CAD build for the part. Positions are in the model's coordinates, mm. Face numbers are marked on the shaded views. A direction names the side the tool comes from. Give positions to 0.01 mm unless a question says otherwise; leave off trailing zeros. Write each loop counter-clockwise with the first axis right and the second up, starting at its lowest first coordinate (ties: lowest second). Pieces come first, ordered by that corner, then holes. Notation, with made-up numbers: (-39.75, 14.25) - (-29.75, 14.25) arc R25 ccw to (-29.75, 47.25) - close; hole circle Ø9 at (-2, 22.5). An arc over 180 degrees is marked (long way). Answer as a JSON object with one key per item and string values.
from build123d import *

# Parameters (mm, degrees)
F1_DEPTH  = 10
F3_DEPTH  = 100
F4_R      = 35
F5_DEPTH  = 90
F6_DEPTH  = 95.001
F7_R      = 5
F10_R     = 4
F11_DEPTH = 18


with BuildPart() as f1:
    # F0 (on Top) → F1 (new body)
    with BuildSketch(Plane.XY):
        Polygon((-6, 61.6815258077), (-6, 41.6815258077), (-37, 41.6815258077), (-37, 29.6815258077), (-28.3371814517, 29.6815258077), (-40, -30.3184741923), (-40, -125.3184741923), (0, -125.3184741923), (40, -125.3184741923), (40, -30.3184741923), (28.3371814517, 29.6815258077), (37, 29.6815258077), (37, 41.6815258077), (6, 41.6815258077), (6, 61.6815258077), (0, 61.6815258077), align=None)
        Polygon((-8.5239209836, -30.3184741923), (-32, -30.3184741923), (-22.8734250069, 16.6336838404), align=None, mode=Mode.SUBTRACT)
        Polygon((-18.3371814517, 29.6815258077), (-6, 29.6815258077), (-6, -10.686231312), align=None, mode=Mode.SUBTRACT)
        Polygon((6, -10.686231312), (6, 29.6815258077), (18.3371814517, 29.6815258077), align=None, mode=Mode.SUBTRACT)
        Polygon((22.8734250069, 16.6336838404), (32, -30.3184741923), (8.5239209836, -30.3184741923), align=None, mode=Mode.SUBTRACT)
    extrude(amount=F1_DEPTH)

    # F2 (on face) → F3 (join)
    with BuildSketch(Plane.XY.offset(10)):
        Polygon((-8.5239209836, -30.3184741923), (-40, -30.3184741923), (-40, -125.3184741923), (40, -125.3184741923), (40, -30.3184741923), (8.5239209836, -30.3184741923), align=None)
    extrude(amount=F3_DEPTH)

    # F4 (on face) → F5 (cut)
    with BuildSketch(Plane(origin=(0, -30.3184741923, 0), x_dir=(-1, 0, 0), z_dir=(0, 1, 0))):
        with Locations((0, 55)):
            Circle(F4_R)
    extrude(amount=-F5_DEPTH, mode=Mode.SUBTRACT)

    # F4 (on face) → F6 (cut, through all)
    with BuildSketch(Plane(origin=(0, -30.3184741923, 0), x_dir=(-1, 0, 0), z_dir=(0, 1, 0))):
        with BuildLine():
            ThreePointArc((-40, 55), (0, 95), (40, 55))
            Line((40, 55), (40, 110))
            Line((40, 110), (-40, 110))
            Line((-40, 110), (-40, 55))
        make_face()
    extrude(amount=-F6_DEPTH, mode=Mode.SUBTRACT)

    # F7
    f7_edges = [f1.edges().sort_by_distance(p)[0] for p in [
        (0, -30.318474, 10),
        (-8.523921, -30.318474, 5),
        (8.523921, -30.318474, 5),
        (36, -30.318474, 10),
        (32, -30.318474, 5),
        (-36, -30.318474, 10),
        (-32, -30.318474, 5),
    ]]
    fillet(f7_edges, radius=F7_R)

    # F10 (on face) → F11 (cut)
    with BuildSketch(Plane(origin=(0, 7.9203814519, 13.7185030901), x_dir=(1, 0, 0), z_dir=(0, 0.5, 0.8660254038))):
        with Locations((0, 44.4177682936)):
            Circle(F10_R)
    extrude(amount=F11_DEPTH, mode=Mode.SUBTRACT)


solid = f1.part
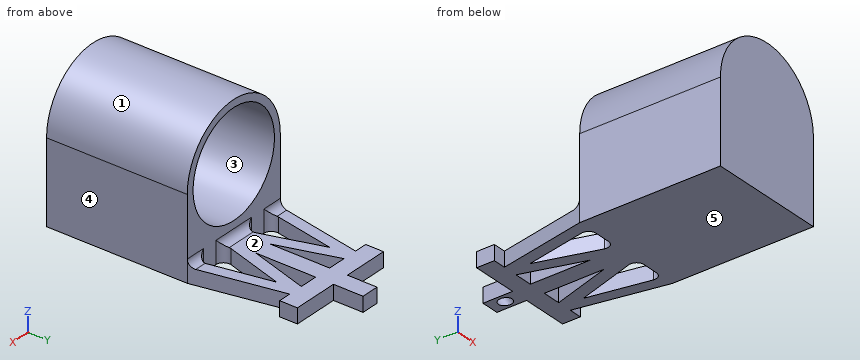
(1) Saw through at D-D, the plane x = 0. Give the cut face in (y, z).
Answer key:
{"outline": "(-125.32, 0) - (46.67, 0) - (51.92, 9.1) - (58.85, 5.1) - (55.91, 0) - (61.68, 0) - (61.68, 10) - (-25.32, 10) arc R5 cw to (-30.32, 15) - (-30.32, 20) - (-120.32, 20) - (-120.32, 90) - (-30.32, 90) - (-30.32, 95) - (-125.32, 95) - close"}
(2) Saw through at B-B, the plane y = 2.5. Give the cut face in (x, z), and give its area (3 significant figures).
Answer key:
{"outline": "(-33.62, 0) - (-25.62, 0) - (-25.62, 10) - (-33.62, 10) - close; (-18.55, 0) - (-10.03, 0) - (-10.03, 10) - (-18.55, 10) - close; (-6, 0) - (6, 0) - (6, 10) - (-6, 10) - close; (10.03, 0) - (18.55, 0) - (18.55, 10) - (10.03, 10) - close; (25.62, 0) - (33.62, 0) - (33.62, 10) - (25.62, 10) - close", "area": "450 mm²"}
(3) Flat gauge pins, fed straight in: P1, Ø5, axis at x = -18.5, z = 7, coming from the +Y side; P2, Ø3, axis at y = 48, z = 3.5, coming from the -X side; P3, Ø3, axis at y = 17, z = 5.5, coming from the -X side. Where does each tip first touch, or does it go through?
Answer key:
{"P1": "stops at y = 41.68", "P2": "stops at x = -6", "P3": "stops at x = -31.09"}
(4) Probe L1, parallel to Z at x = 0, y = -82; L2, parallel to Y at x = 6.5, z = 63; L3, parallel to Z at x = -18.5, y = -69.5. List the from-to ranges inside material, lowest first. Write a range as [from, to].
Answer key:
{"L1": "z = [0, 20], [90, 95]", "L2": "y = [-125.32, -120.32]", "L3": "z = [0, 25.29], [84.71, 90.46]"}
(5) 3-axis set-ups, long thin cutter, end or side, ignore diameter. For the marked faces 1 and 2: which of +Z, -Z, +X, -X, +Y, -Y reach the whole face in a straight line?
Answer key:
{"face 1": "+Z, +Y, -Y", "face 2": "+Z, +X, -X, +Y"}
(6) Pull direction X, two halves, no side cores. Call the marked faces 3, 4 and 5: pulls with the +X half, pulls with the -X half, needs draft (parallel to the pull), parting line crosses it, or undercut.
Answer key:
{"face 3": "undercut", "face 4": "pulls with the +X half", "face 5": "needs draft"}
(7) Saw through at C-C, the plane z = 23. Give the cut face in (x, y), and give its area (3 significant figures).
Answer key:
{"outline": "(-40, -125.32) - (40, -125.32) - (40, -30.32) - (14.18, -30.32) - (14.18, -120.32) - (-14.18, -120.32) - (-14.18, -30.32) - (-40, -30.32) - close", "area": "5,050 mm²"}
(8) Saw through at A-A, the plane y = -84. Give the cut face in (x, z).
Answer key:
{"outline": "(-40, 0) - (40, 0) - (40, 55) arc R40 ccw to (-40, 55) - close; hole circle Ø70 at (0, 55)"}
